Could you check a few things on this model? Use its own coordinates, in mm. Face numbers are marked on the shaded views. Give positions to 0.01 mm unless a question says otherwise; leave off trailing zeros. Loops run counter-clockwise (first coordinate to the right, second up) from the corner with the lowest first, then second, coordinate; pieces in that order, holes last. Notation, with made-up numbers: M 86.5,66.5 L 102.5,66.5 A16 ccw 102.5,96.5 Z; hole C 61.25,29 d9. An arc over 180 degrees is marked long. Answer in a Markdown table with one row per item. Add a question column.
```python
from build123d import *

# Parameters (mm, degrees)
F1_DEPTH = 30
F2_DEPTH = 15
F3_R     = 1
F4_R     = 1
F5_SIZE  = 1


with BuildPart() as f1:
    # F0 (on Top) → F1 (new body)
    with BuildSketch(Plane.XY):
        with BuildLine():
            Line((-6.0564657358, 20.029321317), (-102.5407865696, 20.029321317))
            ThreePointArc((-102.5407865696, 20.029321317), (-98.9986261527, 15.029321317), (-102.5407865696, 10.029321317))
            Line((-102.5407865696, 10.029321317), (-6.0564657358, 10.029321317))
            ThreePointArc((-6.0564657358, 10.029321317), (-9.5986261527, 15.029321317), (-6.0564657358, 20.029321317))
        make_face()
    extrude(amount=F1_DEPTH)

    # F0 (on Top) → F2 (join)
    with BuildSketch(Plane.XY):
        with BuildLine():
            Line((-104.2986261527, 17.529321317), (-104.2986261527, 20.029321317))
            ThreePointArc((-104.2986261527, 20.029321317), (-109.2986261527, 15.029321317), (-104.2986261527, 10.029321317))
            Line((-104.2986261527, 10.029321317), (-104.2986261527, 12.529321317))
            ThreePointArc((-104.2986261527, 12.529321317), (-106.7986261527, 15.029321317), (-104.2986261527, 17.529321317))
        make_face()
        with BuildLine():
            Line((-102.5407865696, 20.029321317), (-104.2986261527, 20.029321317))
            Line((-104.2986261527, 20.029321317), (-104.2986261527, 17.529321317))
            ThreePointArc((-104.2986261527, 17.529321317), (-102.5308591998, 16.7970882699), (-101.7986261527, 15.029321317))
            ThreePointArc((-101.7986261527, 15.029321317), (-102.5308591998, 13.261554364), (-104.2986261527, 12.529321317))
            Line((-104.2986261527, 12.529321317), (-104.2986261527, 10.029321317))
            Line((-104.2986261527, 10.029321317), (-102.5407865696, 10.029321317))
            ThreePointArc((-102.5407865696, 10.029321317), (-98.9986261527, 15.029321317), (-102.5407865696, 20.029321317))
        make_face()
        with BuildLine():
            ThreePointArc((-4.2986261527, 10.029321317), (0.7013738473, 15.029321317), (-4.2986261527, 20.029321317))
            Line((-4.2986261527, 20.029321317), (-4.2986261527, 17.529321317))
            ThreePointArc((-4.2986261527, 17.529321317), (-2.5308591998, 16.7970882699), (-1.7986261527, 15.029321317))
            ThreePointArc((-1.7986261527, 15.029321317), (-2.5308591998, 13.261554364), (-4.2986261527, 12.529321317))
            Line((-4.2986261527, 12.529321317), (-4.2986261527, 10.029321317))
        make_face()
        with BuildLine():
            Line((-4.2986261527, 20.029321317), (-6.0564657358, 20.029321317))
            ThreePointArc((-6.0564657358, 20.029321317), (-9.5986261527, 15.029321317), (-6.0564657358, 10.029321317))
            Line((-6.0564657358, 10.029321317), (-4.2986261527, 10.029321317))
            Line((-4.2986261527, 10.029321317), (-4.2986261527, 12.529321317))
            ThreePointArc((-4.2986261527, 12.529321317), (-6.7986261527, 15.029321317), (-4.2986261527, 17.529321317))
            Line((-4.2986261527, 17.529321317), (-4.2986261527, 20.029321317))
        make_face()
    extrude(amount=F2_DEPTH)

    # F3
    f3_edges = [f1.edges().sort_by_distance(p)[0] for p in [
        (-102.540787, 20.029321, 22.5),
        (-102.540787, 10.029321, 22.5),
        (-6.056466, 20.029321, 22.5),
        (-6.056466, 10.029321, 22.5),
    ]]
    fillet(f3_edges, radius=F3_R)

    # F4
    f4_edges = [f1.edges().sort_by_distance(p)[0] for p in [
        (-54.298626, 20.029321, 30),
        (-54.298626, 10.029321, 0),
    ]]
    fillet(f4_edges, radius=F4_R)

    # F5
    f5_edges = [f1.edges().sort_by_distance(p)[0] for p in [
        (-104.298626, 12.529321, 0),
        (-4.298626, 17.529321, 0),
    ]]
    chamfer(f5_edges, length=F5_SIZE)


solid = f1.part
```
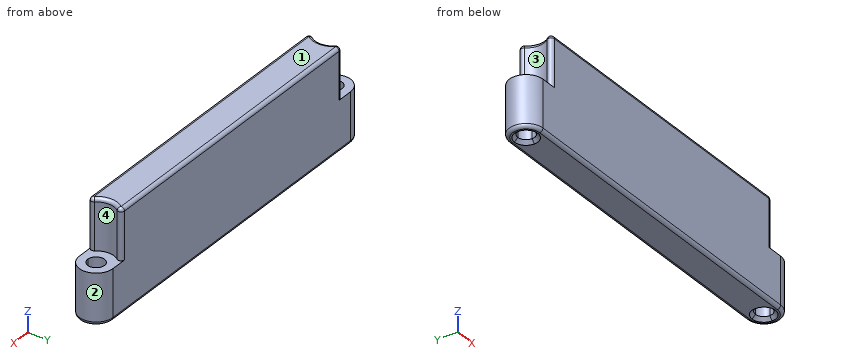
Item 1: For P1, Ø3, axis at x = -102.5, y = 17.5, coming from the +Z side, with a flat end and sliding along its axis, tell me the tip position at first contact or that it passes through.
Item 2: Suppose I cut it at B-B (z = 17.75). List the corners of the cut face in (x, y) for me.
Item 3: Suppose I cut it at C-C (y = 16). Give the number of separate pieces and of enclosed holes in the cut face, then the cut area to 3 significant figures.
Item 4: Suppose I cut it at A-A (z = 7.75). List the corners of the cut face in (x, y) for me.
Item 5: I need wall thicknesses on L1, parallel to X at y = 15.5, z = 7.5; L2, parallel to X at y = 14.5, z = 12.25; L3, parallel to Z at x = -9, y = 16. Which ranges of each line are inside material? Lowest first, please.
Item 6: If we mould it in two halves opening along Y, with no side actions, what happens to the marked faces 1, 2, 3 and 4? For each: +Y half, -Y half, draft (parallel to the pull), parting line (faces both ways), or undercut.
Values found:
| question | item | result |
|---|---|---|
| 1 | P1 | z = 15 |
| 2 | outline | M -100.2,11.66 A1 ccw -99.43,10.03 L -9.17,10.03 A1 ccw -8.39,11.66 A5.3 cw -8.39,18.39 A1 ccw -9.17,20.03 L -99.43,20.03 A1 ccw -100.2,18.39 A5.3 cw Z |
| 3 | separate pieces | 3 |
| 3 | enclosed holes | 0 |
| 3 | area | 2,850 mm² |
| 4 | outline | M -104.3,10.03 L -4.3,10.03 A5 ccw -4.3,20.03 L -104.3,20.03 A5 ccw Z; hole C -104.3,15.03 d5; hole C -4.3,15.03 d5 |
| 5 | L1 | -109.28 to -106.75, -101.84 to -6.75, -1.84 to 0.68 |
| 5 | L2 | -109.27 to -106.74, -101.86 to -6.74, -1.86 to 0.67 |
| 5 | L3 | 0 to 15 |
| 6 | face 1 | draft |
| 6 | face 2 | parting line |
| 6 | face 3 | undercut |
| 6 | face 4 | undercut |
